The model under review builds one solid part; all positions refer to its coordinate system, in mm. Face numbers are marked on the shaded views. A direction names the side the tool comes from. Round coordinates to 2 decimals unless told otherwise and drop trailing zeros. Write each loop counter-clockwise with the first axis right and the second up, starting at its lowest first coordinate (ties: lowest second). Pieces come first, ordered by that corner, then holes. Notation, with made-up numbers: (30.5, -1) -> (56.5, -1) arc R21 cw to (56.5, 10) -> close; hole circle Ø6 at (-22.75, -22). An arc over 180 degrees is marked (long way). Use CSV: the item, a comma, the result in double quotes. Start each with the question number.
1) Take a section at D-D, the plane x = -9. Give the boundary of the cut face in (y, z).
2) Machinability: for the marked faces 1 and 2, which of the approach directions +Z, -Z, +X, -X, +Y, -Y give a long, thin tool a straight path to every point of the face, cutting with its end or side? Answer none if there is none.
3) Mouldability with a two-part tool opening along X and no side actions: class the marked faces 3, 4 and 5 as released by +X, released by -X, zero draft, split by the parting line, or undercut.
4) Wall thickness on probe 1 along Y at (x, z) = (0, 4); probe 2 along Y at (x, z) = (-2, 10.5); probe 3 along X at (y, z) = (-10, 2.5): over which ranges is each line inside the solid? List them lowest first. Write a range as [from, to].
5) Take a section at A-A, the plane x = 0. Give the boundary of the cut face in (y, z), then the cut area to 3 significant figures.
6) For pin 1 Ø1 at (y, z) = (-6, 8.5) entering from +X; pin 2 Ø6.5 at (y, z) = (-7, 4) entering from -X; pin 3 Ø3 at (x, z) = (-8.5, 10) entering from -Y, all flat-tipped, find the tip position at first contact; note any pin that passes through.
7) Take a section at C-C, the plane z = 4. Give the boundary of the cut face in (x, y).
8) Take a section at B-B, the plane y = 0. Give the boundary of the cut face in (x, z).
from build123d import *

# Parameters (mm, degrees)
F0_R     = 22.5
F1_DEPTH = 10
F3_R     = 19.5
F4_DEPTH = 2
F5_R     = 2.65
F5_W     = 27
F5_H     = 8
F6_DEPTH = 12.001
F8_R     = 1


with BuildPart() as f1:
    # F0 (on Top) → F1 (new body)
    with BuildSketch(Plane.XY):
        Circle(F0_R)
    extrude(amount=F1_DEPTH)

    # F3 (on face) → F4 (join)
    with BuildSketch(Plane.XY.offset(10)):
        Circle(F3_R)
    extrude(amount=F4_DEPTH)

    # F5 (on face) → F6 (cut, through all)
    with BuildSketch(Plane.XY.offset(12)):
        Circle(F5_R)
        with Locations((0, -8.5)):
            Rectangle(F5_W, F5_H)
    extrude(amount=-F6_DEPTH, mode=Mode.SUBTRACT)

    # F8
    f8_edges = [f1.edges().sort_by_distance(p)[0] for p in [
        (-13.5, -12.5, 6),
        (-13.5, -4.5, 6),
        (13.5, -4.5, 6),
        (13.5, -12.5, 6),
    ]]
    fillet(f8_edges, radius=F8_R)


solid = f1.part
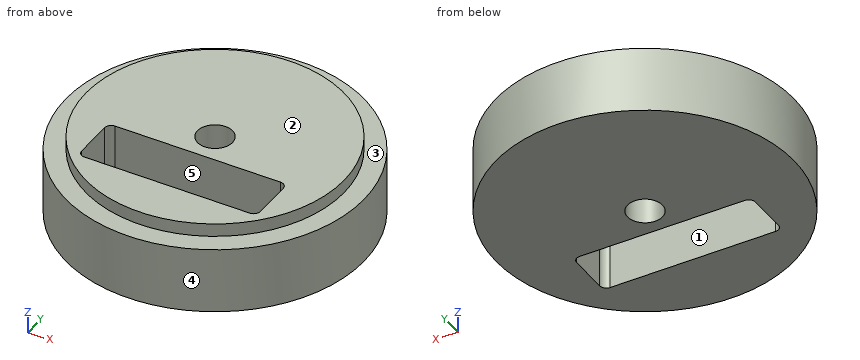
Values found:
1,outline,"(-20.62, 0) -> (-12.5, 0) -> (-12.5, 12) -> (-17.3, 12) -> (-17.3, 10) -> (-20.62, 10) -> close; (-4.5, 0) -> (20.62, 0) -> (20.62, 10) -> (17.3, 10) -> (17.3, 12) -> (-4.5, 12) -> close"
2,face 1,"+Z, -Z"
2,face 2,"+Z, +X, -X, +Y, -Y"
3,face 3,"zero draft"
3,face 4,"split by the parting line"
3,face 5,"undercut"
4,probe 1,"[-22.5, -12.5], [-4.5, -2.65], [2.65, 22.5]"
4,probe 2,"[-19.4, -12.5], [-4.5, -1.74], [1.74, 19.4]"
4,probe 3,"[-20.16, -13.5], [13.5, 20.16]"
5,outline,"(-22.5, 0) -> (-12.5, 0) -> (-12.5, 12) -> (-19.5, 12) -> (-19.5, 10) -> (-22.5, 10) -> close; (-4.5, 0) -> (-2.65, 0) -> (-2.65, 12) -> (-4.5, 12) -> close; (2.65, 0) -> (22.5, 0) -> (22.5, 10) -> (19.5, 10) -> (19.5, 12) -> (2.65, 12) -> close"
5,area,"368 mm²"
6,pin 1,"x = 21.82"
6,pin 2,"x = -22.19"
6,pin 3,"y = -21.38"
7,outline,"circle Ø45 at (0, 0); hole (-13.5, -11.5) arc R1 ccw to (-12.5, -12.5) -> (12.5, -12.5) arc R1 ccw to (13.5, -11.5) -> (13.5, -5.5) arc R1 ccw to (12.5, -4.5) -> (-12.5, -4.5) arc R1 ccw to (-13.5, -5.5) -> close; hole circle Ø5.3 at (0, 0)"
8,outline,"(-22.5, 0) -> (-2.65, 0) -> (-2.65, 12) -> (-19.5, 12) -> (-19.5, 10) -> (-22.5, 10) -> close; (2.65, 0) -> (22.5, 0) -> (22.5, 10) -> (19.5, 10) -> (19.5, 12) -> (2.65, 12) -> close"
